For this review, use the dimensioned drawing (mm, ordinates from the lowest corner) and the shaded views. A direction names the side the tool comes from. Coordinates: 2 decimals unless noted, no trailing zeros. Order: outer loops, then holes, each group sorted by start corner. A loop starts at its lowest first (then second) coordinate and runs counter-clockwise, first axis right, second up. Notation, with made-up numbers: (42.25, 53) -> (73.25, 53) arc R16 ccw to (73.25, 68) -> close; hole circle Ø7 at (0.25, 25.25). An arc over 180 degrees is marked (long way). Return JSON: item names as keys, results as strings. Group by question number.
Item 1: Draft analysis for pull direction Z (two halves, no side actions). For the marked faces 1, 2 and 3, state which applies: +Z half, -Z half, draft (parallel to the pull), parting line (faces both ways), or undercut.
Item 2: Take a section at D-D (x = 15). Write out the cut boundary in (y, z), then the cut area to 4 significant figures.
Item 3: For line 1 along Z through (x, y) = (6.5, 14); line 2 along Y through (x, z) = (3, 12); line 3 along Y through (x, z) = (27.2, 7.25), list the stretches that pass through material, from the lowest coordinate up.
Item 4: Take a section at B-B (z = 15.5). Write out the cut boundary in (x, y), then the cut area to 3 significant figures.
Item 5: Insertion check: pin 1 (3.5 mm diameter, centred on x = 2.8, y = 2.8, fed in from +Z); pin 2 (3 mm diameter, centred on x = 17.5, z = 36.5, fed in from -Y); pin 3 (8 mm diameter, centred on x = 11.5, z = 35, fed in from -Y). Each pin has a flat end and moves straight along its axis. Give the tip position at first contact, or say it passes through.
Item 6: Machinability: for the marked faces 4, 5 and 6, which of the approach directions +Z, -Z, +X, -X, +Y, -Y give a long, thin tool a straight path to every point of the face, cutting with its end or side? Answer none if there is none.
Item 7: Take a section at A-A (x = 27.2). Write out the cut boundary in (y, z), then the cut area to 3 significant figures.
Item 8: Take a section at C-C (y = 7). Write out the cut boundary in (x, z).
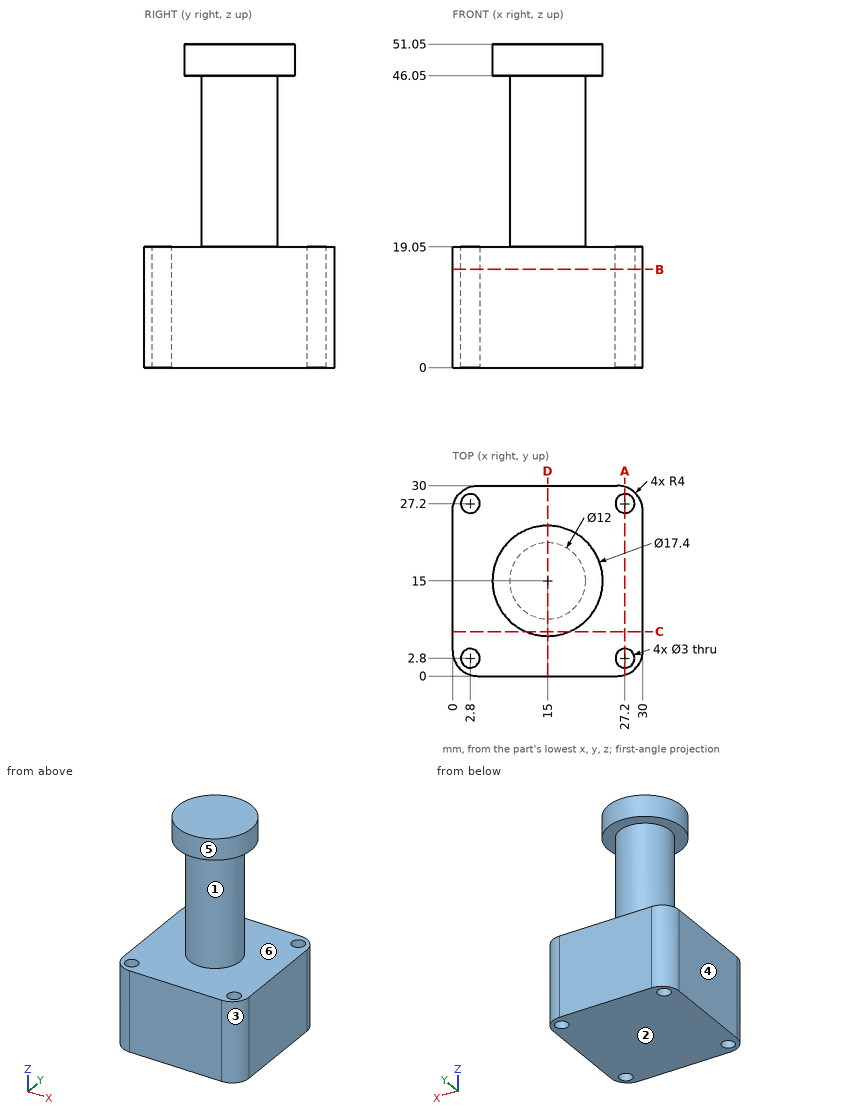
Findings below:
{
 "1": {"face 1": "undercut", "face 2": "-Z half", "face 3": "draft"},
 "2": {"outline": "(0, 0) -> (30, 0) -> (30, 19.05) -> (21, 19.05) -> (21, 46.05) -> (23.7, 46.05) -> (23.7, 51.05) -> (6.3, 51.05) -> (6.3, 46.05) -> (9, 46.05) -> (9, 19.05) -> (0, 19.05) -> close", "area": "982.5 mm2"},
 "3": {"line 1": "z = 0 to 19.05, 46.05 to 51.05", "line 2": "y = 0.13 to 1.31, 4.29 to 25.71, 28.69 to 29.87", "line 3": "y = 0.18 to 1.3, 4.3 to 25.7, 28.7 to 29.82"},
 "4": {"outline": "(0, 4) arc R4 ccw to (4, 0) -> (26, 0) arc R4 ccw to (30, 4) -> (30, 26) arc R4 ccw to (26, 30) -> (4, 30) arc R4 ccw to (0, 26) -> close; hole circle Ø3 at (2.8, 2.8); hole circle Ø3 at (2.8, 27.2); hole circle Ø3 at (27.2, 2.8); hole circle Ø3 at (27.2, 27.2)", "area": "858 mm2"},
 "5": {"pin 1": "stops at z = 19.05", "pin 2": "stops at y = 9.08", "pin 3": "stops at y = 9"},
 "6": {"face 4": "+Z, -Z, -X, +Y, -Y", "face 5": "+Z", "face 6": "none"},
 "7": {"outline": "(0.18, 0) -> (1.3, 0) -> (1.3, 19.05) -> (0.18, 19.05) -> close; (4.3, 0) -> (25.7, 0) -> (25.7, 19.05) -> (4.3, 19.05) -> close; (28.7, 0) -> (29.82, 0) -> (29.82, 19.05) -> (28.7, 19.05) -> close", "area": "450 mm2"},
 "8": {"outline": "(0, 0) -> (30, 0) -> (30, 19.05) -> (0, 19.05) -> close; (11.58, 46.05) -> (18.42, 46.05) -> (18.42, 51.05) -> (11.58, 51.05) -> close"}
}
